Verification items for the finished model (mm, model axes). Face numbers are marked on the shaded views. A direction names the side the tool comes from. Give positions to 0.01 mm unless a question says otherwise; leave off trailing zeros. Loops run counter-clockwise (first coordinate to the right, second up) from the corner with the lowest first, then second, coordinate; pieces in that order, holes last. Notation, with made-up numbers: M 26.5,-0.5 L 52.5,-0.5 A24 ccw 52.5,37.5 Z; hole C -23,-25.5 d9. An arc over 180 degrees is marked long. Use a Markdown table: item, result.
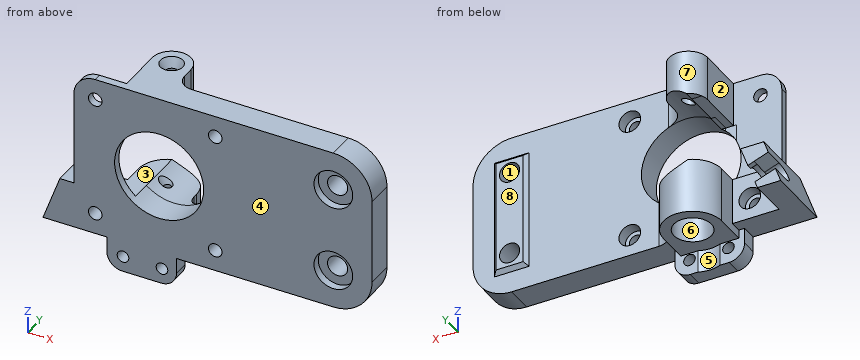
from build123d import *

# Parameters (mm, degrees)
SKETCH1_W                = 77
SKETCH1_H                = 42
BOSS_EXTRUDE1_DEPTH      = 7
FILLET1_R                = 10
FILLET2_R                = 10
FILLET3_R                = 5.5
SKETCH2_W                = 9
SKETCH2_H                = 31
BOSS_EXTRUDE2_DEPTH      = 1
CUT_EXTRUDE1_DEPTH       = 11
CUT_EXTRUDE2_DEPTH       = 31
SKETCH5_R                = 2.6
CUT_EXTRUDE3_DEPTH       = 6
SKETCH6_R                = 2.8
CUT_EXTRUDE4_DEPTH       = 3
SKETCH7_R                = 1.75
CUT_EXTRUDE5_DEPTH       = 4
SKETCH8_W                = 14.5
SKETCH8_H                = 30
CUT_EXTRUDE6_DEPTH       = 5
BOSS_EXTRUDE3_DEPTH      = 11.5
BOSS_EXTRUDE4_DEPTH      = 4
BOSS_EXTRUDE5_DEPTH      = 14.2
FILLET4_R                = 4
FILLET5_R                = 4
SKETCH12_R               = 11.5
CUT_EXTRUDE7_DEPTH       = 14
CUT_EXTRUDE7_DEPTH_BACK  = 14
SKETCH13_W               = 6.185296294
SKETCH13_H               = 18.5
CUT_EXTRUDE8_DEPTH       = 14
BOSS_EXTRUDE6_DEPTH      = 10
BOSS_EXTRUDE6_DEPTH_BACK = 7
CUT_EXTRUDE9_DEPTH       = 10
SKETCH16_R               = 4.85
CUT_EXTRUDE10_DEPTH      = 10
SKETCH17_R               = 1
CUT_EXTRUDE11_DEPTH      = 5
SKETCH19_R               = 2.8
CUT_EXTRUDE12_DEPTH      = 3
SKETCH20_R               = 1.75
CUT_EXTRUDE13_DEPTH      = 8
SKETCH21_R               = 4.5
CUT_EXTRUDE14_DEPTH      = 1.7
CUT_EXTRUDE15_DEPTH      = 1.7
CUT_EXTRUDE15_DEPTH_BACK = 31.7
SKETCH23_R               = 1.75
CUT_EXTRUDE16_DEPTH      = 50.7
SKETCH24_R               = 2.9
CUT_EXTRUDE17_DEPTH      = 2.325
CUT_EXTRUDE17_TAPER      = 30
CUT_EXTRUDE18_REACH      = 49.675
SKETCH25_R               = 1.557660624
SKETCH26_R               = 7
CUT_EXTRUDE19_DEPTH      = 5.8
SKETCH27_R               = 1.5
CUT_EXTRUDE20_DEPTH      = 5.0000001
SKETCH29_R               = 5
CUT_EXTRUDE21_DEPTH      = 2
MIRROR5_COPY_1_SKETCH_R  = 2.6
MIRROR5_COPY_1_DEPTH     = 6
MIRROR5_COPY_2_SKETCH_R  = 2.6
MIRROR5_COPY_2_DEPTH     = 6
SKETCH35_R               = 1
CUT_EXTRUDE23_DEPTH      = 2.3
CUT_EXTRUDE23_TAPER      = -28


with BuildPart() as part:
    # Sketch1 → Boss-Extrude1 (new body)
    with BuildSketch(Plane(origin=(0, 0, 0), x_dir=(1, 0, 0), z_dir=(0, 1, 0))):
        with Locations((38.5, 21)):
            Rectangle(SKETCH1_W, SKETCH1_H)
    extrude(amount=BOSS_EXTRUDE1_DEPTH)

    # Fillet1
    fillet1_edges = [part.edges().sort_by_distance(p)[0] for p in [
        (77, 3.5, 0),
    ]]
    fillet(fillet1_edges, radius=FILLET1_R)

    # Fillet2
    fillet2_edges = [part.edges().sort_by_distance(p)[0] for p in [
        (77, 3.5, -42),
    ]]
    fillet(fillet2_edges, radius=FILLET2_R)

    # Fillet3
    fillet3_edges = [part.edges().sort_by_distance(p)[0] for p in [
        (0, 3.5, 0),
    ]]
    fillet(fillet3_edges, radius=FILLET3_R)

    # Sketch2 → Boss-Extrude2 (add)
    with BuildSketch(Plane(origin=(0, 7, 0), x_dir=(1, 0, 0), z_dir=(0, 1, 0))):
        with Locations((67, 21)):
            Rectangle(SKETCH2_W, SKETCH2_H)
    extrude(amount=BOSS_EXTRUDE2_DEPTH)

    # Sketch3 → Cut-Extrude1 (cut)
    with BuildSketch(Plane(origin=(71.5, 0, 0), x_dir=(0, 0, -1), z_dir=(1, 0, 0))):
        Polygon((5.5, 7), (5.5, 8), (6.5, 8), align=None)
    cut_extrude1 = extrude(amount=-CUT_EXTRUDE1_DEPTH, mode=Mode.SUBTRACT)

    # Sketch4 → Cut-Extrude2 (cut)
    with BuildSketch(Plane(origin=(0, 0, -36.5), x_dir=(-1, 0, 0), z_dir=(0, 0, -1))):
        Polygon((-71.5, 8), (-70.5, 8), (-71.5, 7), align=None)
        Polygon((-62.5, 8), (-62.5, 7), (-63.5, 8), align=None)
    extrude(amount=-CUT_EXTRUDE2_DEPTH, mode=Mode.SUBTRACT)

    # Mirror2: Cut-Extrude1 across plane
    add(cut_extrude1.mirror(Plane.XY.offset(-21)), mode=Mode.SUBTRACT)

    # Sketch5 → Cut-Extrude3 (cut)
    with BuildSketch(Plane(origin=(0, 8, 0), x_dir=(1, 0, 0), z_dir=(0, 1, 0))):
        with Locations((67, 10)):
            Circle(SKETCH5_R)
    cut_extrude3 = extrude(amount=-CUT_EXTRUDE3_DEPTH, mode=Mode.SUBTRACT)

    # Mirror3: Cut-Extrude3 across plane
    add(cut_extrude3.mirror(Plane.XY.offset(-21)), mode=Mode.SUBTRACT)

    # Sketch6 → Cut-Extrude4 (cut)
    with BuildSketch(Plane(origin=(0, 7, 0), x_dir=(1, 0, 0), z_dir=(0, 1, 0))):
        with Locations((36.5, 5.5)):
            Circle(SKETCH6_R)
    cut_extrude4 = extrude(amount=-CUT_EXTRUDE4_DEPTH, mode=Mode.SUBTRACT)

    # Sketch7 → Cut-Extrude5 (cut)
    with BuildSketch(Plane(origin=(0, 4, 0), x_dir=(1, 0, 0), z_dir=(0, 1, 0))):
        with Locations((36.5, 5.5)):
            Circle(SKETCH7_R)
    cut_extrude5 = extrude(amount=-CUT_EXTRUDE5_DEPTH, mode=Mode.SUBTRACT)

    # Mirror4: Cut-Extrude4, Cut-Extrude5 across plane
    add(cut_extrude4.mirror(Plane.XY.offset(-21)), mode=Mode.SUBTRACT)
    add(cut_extrude5.mirror(Plane.XY.offset(-21)), mode=Mode.SUBTRACT)

    # Sketch8 → Cut-Extrude6 (cut)
    with BuildSketch(Plane(origin=(0, 7, 0), x_dir=(1, 0, 0), z_dir=(0, 1, 0))):
        with Locations((7.25, 15)):
            Rectangle(SKETCH8_W, SKETCH8_H)
    extrude(amount=-CUT_EXTRUDE6_DEPTH, mode=Mode.SUBTRACT)

    # Sketch9 → Boss-Extrude3 (add)
    with BuildSketch(Plane.XY):
        with BuildLine():
            Line((12.5, 2), (12.5, 14))
            ThreePointArc((12.5, 14), (17.5, 19), (22.5, 14))
            Line((22.5, 14), (22.5, 7))
            Line((22.5, 7), (14.5, 7))
            Line((14.5, 7), (14.5, 2))
            Line((14.5, 2), (12.5, 2))
        make_face()
    extrude(amount=-BOSS_EXTRUDE3_DEPTH)

    # Sketch10 → Boss-Extrude4 (add)
    with BuildSketch(Plane.XZ):
        with BuildLine():
            Line((26.5, -42), (26.5, -46))
            ThreePointArc((26.5, -46), (25.328427125, -48.828427125), (22.5, -50))
            Line((22.5, -50), (12.5, -50))
            ThreePointArc((12.5, -50), (9.671572875, -48.828427125), (8.5, -46))
            Line((8.5, -46), (8.5, -42))
            Line((8.5, -42), (26.5, -42))
        make_face()
    extrude(amount=-BOSS_EXTRUDE4_DEPTH)

    # Sketch11 → Boss-Extrude5 (add)
    with BuildSketch(Plane(origin=(0, 0, -44.2), x_dir=(-1, 0, 0), z_dir=(0, 0, -1))):
        with BuildLine():
            Line((-25, 4), (-25, 12))
            ThreePointArc((-25, 12), (-17.5, 19.5), (-10, 12))
            Line((-10, 12), (-10, 4))
            Line((-10, 4), (-25, 4))
        make_face()
    extrude(amount=-BOSS_EXTRUDE5_DEPTH)

    # Fillet4
    fillet4_edges = [part.edges().sort_by_distance(p)[0] for p in [
        (22.5, 7, -5.75),
    ]]
    fillet(fillet4_edges, radius=FILLET4_R)

    # Fillet5
    fillet5_edges = [part.edges().sort_by_distance(p)[0] for p in [
        (25, 7, -36),
    ]]
    fillet(fillet5_edges, radius=FILLET5_R)

    # Sketch12 → Cut-Extrude7 (cut, two sides)
    with BuildSketch(Plane(origin=(0, 7, 0), x_dir=(1, 0, 0), z_dir=(0, 1, 0))) as cut_extrude7_sk:
        with Locations((22, 21)):
            Circle(SKETCH12_R)
    extrude(amount=CUT_EXTRUDE7_DEPTH, mode=Mode.SUBTRACT)
    extrude(cut_extrude7_sk.sketch, amount=-CUT_EXTRUDE7_DEPTH_BACK, mode=Mode.SUBTRACT)

    # Sketch13 → Cut-Extrude8 (cut)
    with BuildSketch(Plane(origin=(0, 2, 0), x_dir=(1, 0, 0), z_dir=(0, 1, 0))):
        with Locations((14.723239075, 20.75)):
            Rectangle(SKETCH13_W, SKETCH13_H)
    extrude(amount=CUT_EXTRUDE8_DEPTH, mode=Mode.SUBTRACT)

    # Sketch14 → Boss-Extrude6 (add, two sides)
    with BuildSketch(Plane(origin=(0, 7, 0), x_dir=(1, 0, 0), z_dir=(0, 1, 0))) as boss_extrude6_sk:
        Polygon((10, 42), (-8, 42), (-3.632357189, 30), (10, 30), align=None)
    extrude(amount=BOSS_EXTRUDE6_DEPTH)
    extrude(boss_extrude6_sk.sketch, amount=-BOSS_EXTRUDE6_DEPTH_BACK)

    # Sketch15 → Cut-Extrude9 (cut)
    with BuildSketch(Plane(origin=(0, 17, 0), x_dir=(1, 0, 0), z_dir=(0, 1, 0))):
        Polygon((10, 42), (10, 30), (2.367642811, 30), (-2, 42), align=None)
    extrude(amount=-CUT_EXTRUDE9_DEPTH, mode=Mode.SUBTRACT)

    # Sketch16 → Cut-Extrude10 (cut)
    with BuildSketch(Plane(origin=(0, 0, -44.2), x_dir=(-1, 0, 0), z_dir=(0, 0, -1))):
        with Locations((-17.5, 12)):
            Circle(SKETCH16_R)
    extrude(amount=-CUT_EXTRUDE10_DEPTH, mode=Mode.SUBTRACT)

    # Sketch17 → Cut-Extrude11 (cut)
    with BuildSketch(Plane(origin=(0, 0, -34.2), x_dir=(-1, 0, 0), z_dir=(0, 0, -1))):
        with Locations((-17.5, 12)):
            Circle(SKETCH17_R)
    extrude(amount=-CUT_EXTRUDE11_DEPTH, mode=Mode.SUBTRACT)

    # Sketch19 → Cut-Extrude12 (cut)
    with BuildSketch(Plane(origin=(0, 7, 0), x_dir=(1, 0, 0), z_dir=(0, 1, 0))):
        with Locations((5.5, 36.5)):
            Circle(SKETCH19_R)
    extrude(amount=-CUT_EXTRUDE12_DEPTH, mode=Mode.SUBTRACT)

    # Sketch20 → Cut-Extrude13 (cut)
    with BuildSketch(Plane(origin=(0, 4, 0), x_dir=(1, 0, 0), z_dir=(0, 1, 0))):
        with Locations((5.5, 36.5)):
            Circle(SKETCH20_R)
    extrude(amount=-CUT_EXTRUDE13_DEPTH, mode=Mode.SUBTRACT)

    # Sketch21 → Cut-Extrude14 (cut)
    with BuildSketch(Plane(origin=(11.73249536, 0, -4.270279085), x_dir=(-0.342020143, 0, -0.939692621), z_dir=(0.939692621, 0, -0.342020143))):
        with Locations((35.53099709, 12)):
            Circle(SKETCH21_R)
    extrude(amount=-CUT_EXTRUDE14_DEPTH, mode=Mode.SUBTRACT)

    # Sketch22 → Cut-Extrude15 (cut, two sides)
    with BuildSketch(Plane(origin=(10.135017905, 0, -3.688844841), x_dir=(-0.342020143, 0, -0.939692621), z_dir=(0.939692621, 0, -0.342020143))) as cut_extrude15_sk:
        with BuildLine():
            Line((32.83099709, 12), (32.83099709, 17))
            Line((32.83099709, 17), (38.23099709, 17))
            Line((38.23099709, 17), (38.23099709, 12))
            ThreePointArc((38.23099709, 12), (35.53099709, 9.3), (32.83099709, 12))
        make_face()
    extrude(amount=CUT_EXTRUDE15_DEPTH, mode=Mode.SUBTRACT)
    extrude(cut_extrude15_sk.sketch, amount=-CUT_EXTRUDE15_DEPTH_BACK, mode=Mode.SUBTRACT)

    # Sketch23 → Cut-Extrude16 (cut)
    with BuildSketch(Plane(origin=(0, 2, 0), x_dir=(1, 0, 0), z_dir=(0, 1, 0))):
        with Locations((5.5, 5.5)):
            Circle(SKETCH23_R)
    extrude(amount=-CUT_EXTRUDE16_DEPTH, mode=Mode.SUBTRACT)

    # Sketch24 → Cut-Extrude17 (cut)
    with BuildSketch(Plane.XY):
        with Locations((17.5, 14)):
            Circle(SKETCH24_R)
    extrude(amount=-CUT_EXTRUDE17_DEPTH, taper=CUT_EXTRUDE17_TAPER, mode=Mode.SUBTRACT)

    # Sketch25 → Cut-Extrude18 (cut, up to next)
    with BuildSketch(Plane.XY.offset(-2.325), mode=Mode.PRIVATE) as cut_extrude18_sk1:
        with Locations((17.5, 14)):
            Circle(SKETCH25_R)
    cut_extrude18_tool1 = extrude(cut_extrude18_sk1.sketch, amount=-CUT_EXTRUDE18_REACH, mode=Mode.PRIVATE) & part.part
    add(cut_extrude18_tool1.solids().sort_by_distance((17.5, 14, -2.325))[0], mode=Mode.SUBTRACT)

    # Sketch26 → Cut-Extrude19 (cut)
    with BuildSketch(Plane(origin=(0, 0, -50), x_dir=(-1, 0, 0), z_dir=(0, 0, -1))):
        with Locations((-17.699941677, 10.4)):
            Circle(SKETCH26_R)
    extrude(amount=-CUT_EXTRUDE19_DEPTH, mode=Mode.SUBTRACT)

    # Sketch27 → Cut-Extrude20 (cut, through all)
    with BuildSketch(Plane(origin=(0, 4, 0), x_dir=(1, 0, 0), z_dir=(0, 1, 0))):
        with Locations((22.735431052, 46)):
            Circle(SKETCH27_R)
        with Locations((12.664452301, 46)):
            Circle(SKETCH27_R)
    extrude(amount=-CUT_EXTRUDE20_DEPTH, mode=Mode.SUBTRACT)

    # Sketch29 → Cut-Extrude21 (cut)
    with BuildSketch(Plane(origin=(0, 0, 0), x_dir=(-1, 0, 0), z_dir=(0, -1, 0))):
        with Locations((-67, 32)):
            Circle(SKETCH29_R)
    cut_extrude21 = extrude(amount=-CUT_EXTRUDE21_DEPTH, mode=Mode.SUBTRACT)

    # Mirror5: Cut-Extrude21 across plane
    add(cut_extrude21.mirror(Plane.XY.offset(-21)), mode=Mode.SUBTRACT)

    # Mirror5 copy 1 sketch → Mirror5 copy 1 (cut)
    with BuildSketch(Plane(origin=(0, 8, 0), x_dir=(1, 0, 0), z_dir=(0, 1, 0))):
        with Locations((67, 10)):
            Circle(MIRROR5_COPY_1_SKETCH_R)
    extrude(amount=-MIRROR5_COPY_1_DEPTH, mode=Mode.SUBTRACT)

    # Mirror5 copy 2 sketch → Mirror5 copy 2 (cut)
    with BuildSketch(Plane(origin=(0, 8, -42), x_dir=(1, 0, 0), z_dir=(0, 1, 0))):
        with Locations((67, -10)):
            Circle(MIRROR5_COPY_2_SKETCH_R)
    extrude(amount=-MIRROR5_COPY_2_DEPTH, mode=Mode.SUBTRACT)

    # Sketch35 → Cut-Extrude23 (cut)
    with BuildSketch(Plane.XY.offset(-32.5)):
        with Locations((17.5, 12)):
            Circle(SKETCH35_R)
    extrude(amount=CUT_EXTRUDE23_DEPTH, taper=CUT_EXTRUDE23_TAPER, mode=Mode.SUBTRACT)


solid = part.part
(1) Set-up check for the marked faces 1, 2, 3, 4 and 5: record each of +Z, -Z, +X, -X, +Y, -Y from which the full face is reachable in a straight line by a thin tool's end or side.
Results below:
| item | result |
|---|---|
| face 1 | +Y, -Y |
| face 2 | +Z, -X, +Y |
| face 3 | -X, +Y |
| face 4 | +Z, -Z, +X, -X, -Y |
| face 5 | -Z, +Y |
(2) Cross-section at C-C on x = 28. Record the cut outline in (y, z).
Results below:
| item | result |
|---|---|
| outline | M 0,-42 L 7.13,-42 L 7.13,-30.81 L 0,-30.81 Z; M 0,-11.19 L 7,-11.19 L 7,0 L 0,0 Z |
(3) Cross-section at B-B on z = -21. Record the cut outline in (x, y).
Results below:
| item | result |
|---|---|
| outline | M 0,0 L 10.5,0 L 10.5,2 L 0,2 Z; M 33.5,0 L 77,0 L 77,7 L 71.5,7 L 70.5,8 L 63.5,8 L 62.5,7 L 33.5,7 Z |
(4) Gauge pin test, flat ends, axial feed: P1, Ø4, axis at y = 7, z = -36.5, coming from the +X side; P2, Ø1.3, axis at x = 14, y = 17, coming from the -Z side; P3, Ø8.5, axis at x = 67, z = -10, coming from the +Y side. Record the tip position at first contact, or that the pin passes through.
Results below:
| item | result |
|---|---|
| P1 | x = 76.68 |
| P2 | z = -44.2 |
| P3 | y = 8 |
(5) Material ranges on line 1 (Z direction, x = 67, y = 0.55); line 2 (Z direction, x = 36.5, y = 2.65); line 3 (X direction, y = 14, z = -6.5), recorded low to high.
Results below:
| item | result |
|---|---|
| line 1 | -42 to -37, -27 to -15, -5 to 0 |
| line 2 | -42 to -38.25, -34.75 to -7.25, -3.75 to 0 |
| line 3 | 12.5 to 15.94, 19.06 to 22.5 |
(6) Draft check along X on the marked faces 6, 7 and 8. Enter one of: +X half, -X half, draft (parallel to the pull), parting line (faces both ways), or undercut.
Results below:
| item | result |
|---|---|
| face 6 | undercut |
| face 7 | parting line |
| face 8 | draft |
(7) Cross-section at D-D on x = 17.5. Record the cut outline in (y, z) (3 decimals).
Results below:
| item | result |
|---|---|
| outline | M 0,-50 L 3.403,-50 L 3.403,-44.2 L 7.15,-44.2 L 7.15,-34.2 L 11,-34.2 L 11,-32.5 L 10.512,-31.583 L 0,-31.583 Z; M 0,-10.417 L 12.442,-10.417 L 12.442,-2.325 L 11.1,0 L 0,0 Z; M 13,-34.2 L 16.85,-34.2 L 16.85,-44.2 L 19.5,-44.2 L 19.5,-31.583 L 13.488,-31.583 L 13,-32.5 Z; M 15.558,-10.417 L 19,-10.417 L 19,0 L 16.9,0 L 15.558,-2.325 Z |
(8) Cross-section at A-A on x = 36.5. Record the cut outline in (y, z), then the cut area to 3 significant figures.
Results below:
| item | result |
|---|---|
| outline | M 0,-42 L 7,-42 L 7,-39.3 L 4,-39.3 L 4,-38.25 L 0,-38.25 Z; M 0,-34.75 L 4,-34.75 L 4,-33.7 L 7,-33.7 L 7,-8.3 L 4,-8.3 L 4,-7.25 L 0,-7.25 Z; M 0,-3.75 L 4,-3.75 L 4,-2.7 L 7,-2.7 L 7,0 L 0,0 Z |
| area | 232 mm^2 |
